Read the model definition and answer for the solid it produces. Units are mm, in the model's axes. A direction names the side the tool comes from. Coordinates: 2 decimals unless noted, no trailing zeros. Order: outer loops, then holes, each group sorted by start corner. A loop starts at its lowest first (then second) coordinate and runs counter-clockwise, first axis right, second up.
from build123d import *

# Parameters (mm, degrees)
BOSS_EXTRUDE1_DEPTH = 1


with BuildPart() as part:
    # Sketch1 → Boss-Extrude1 (new body)
    with BuildSketch(Plane(origin=(0, 0, 0.6), x_dir=(-1, 0, 0), z_dir=(0, 0, -1))):
        with BuildLine():
            Line((-4, 45.96), (-29.8, 45.96))
            ThreePointArc((-29.8, 45.96), (-32.628427125, 44.788427125), (-33.8, 41.96))
            Line((-33.8, 41.96), (-33.8, 4))
            ThreePointArc((-33.8, 4), (-32.628427125, 1.171572875), (-29.8, 0))
            Line((-29.8, 0), (-4, 0))
            ThreePointArc((-4, 0), (-1.171572875, 1.171572875), (0, 4))
            Line((0, 4), (0, 41.96))
            ThreePointArc((0, 41.96), (-1.171572875, 44.788427125), (-4, 45.96))
        make_face()
        with BuildLine():
            Line((-7.95, 4), (-3.9, 4))
            ThreePointArc((-3.9, 4), (-2.9, 3), (-3.9, 2))
            Line((-3.9, 2), (-29.9, 2))
            ThreePointArc((-29.9, 2), (-30.9, 3), (-29.9, 4))
            Line((-29.9, 4), (-24.95, 4))
            ThreePointArc((-24.95, 4), (-24.596446609, 4.146446609), (-24.45, 4.5))
            Line((-24.45, 4.5), (-8.45, 4.5))
            ThreePointArc((-8.45, 4.5), (-8.303553391, 4.146446609), (-7.95, 4))
        make_face(mode=Mode.SUBTRACT)
        with BuildLine():
            Line((-3.9, 41.96), (-29.9, 41.96))
            ThreePointArc((-29.9, 41.96), (-30.9, 42.96), (-29.9, 43.96))
            Line((-29.9, 43.96), (-3.9, 43.96))
            ThreePointArc((-3.9, 43.96), (-2.9, 42.96), (-3.9, 41.96))
        make_face(mode=Mode.SUBTRACT)
    extrude(amount=-BOSS_EXTRUDE1_DEPTH)


solid = part.part
Q1. Determine the mould class of faces 3 (the cylindrical face through (1.203, 1.141, 1.093)), 4 (the cylindrical face through (2.9, 43, 1.1)), 5 (the flat face through (17, 23, 1.6)), 6 (the flat face through (17, 2, 1)) for opening direction Y: +Y half, -Y half, draft (parallel to the pull), parting line (faces both ways), or undercut.
Q2. Straight lines are drawn through the part: L1, parallel to Y at x = 28, z = 0.85; L2, parallel to Y at x = 19, z = 0.7; L3, parallel to Y at x = 32.5, z = 0.75. For each, find the intervals that lie inside material, in ascending order.
Q3. Which of the six approach directions +Z, -Z, +X, -X, +Y, -Y give full straight-line access (tool end or side, diameter ignored) to faces 1 (the flat face through (17, 23, 0.6)), 2 (the flat face through (17, 4.5, 1))?
Q4. The part is cut by section C-C, the plane x = 16. Determine the outline of the cut face in (y, z).
Q5. The part is cut by section A-A, the plane z = 0.9. Determine the outline of the cut face in (x, y), then the cut area to 3 significant figures.
Q6. The part is cut by section B-B, the plane y = 42.96. Determine the outline of the cut face in (x, z), then the cut area to 3 significant figures.
Computed values:
1. face 3: -Y half
1. face 4: undercut
1. face 5: draft
1. face 6: undercut
2. L1: y = 0 to 2, 4 to 41.96, 43.96 to 45.96
2. L2: y = 0 to 2, 4.5 to 41.96, 43.96 to 45.96
2. L3: y = 1.05 to 44.91
3. face 1: -Z, +X, -X, +Y, -Y
3. face 2: +Z, -Z
4. outline: (0, 0.6) - (2, 0.6) - (2, 1.6) - (0, 1.6) - close; (4.5, 0.6) - (41.96, 0.6) - (41.96, 1.6) - (4.5, 1.6) - close; (43.96, 0.6) - (45.96, 0.6) - (45.96, 1.6) - (43.96, 1.6) - close
5. outline: (0, 4) arc R4 ccw to (4, 0) - (29.8, 0) arc R4 ccw to (33.8, 4) - (33.8, 41.96) arc R4 ccw to (29.8, 45.96) - (4, 45.96) arc R4 ccw to (0, 41.96) - close; hole (3.9, 2) - (29.9, 2) arc R1 ccw to (29.9, 4) - (24.95, 4) arc R0.5 cw to (24.45, 4.5) - (8.45, 4.5) arc R0.5 cw to (7.95, 4) - (3.9, 4) arc R1 ccw to start; hole (3.9, 41.96) - (29.9, 41.96) arc R1 ccw to (29.9, 43.96) - (3.9, 43.96) arc R1 ccw to start
5. area: 1,420 mm2
6. outline: (0.13, 0.6) - (2.9, 0.6) - (2.9, 1.6) - (0.13, 1.6) - close; (30.9, 0.6) - (33.67, 0.6) - (33.67, 1.6) - (30.9, 1.6) - close
6. area: 5.55 mm2
